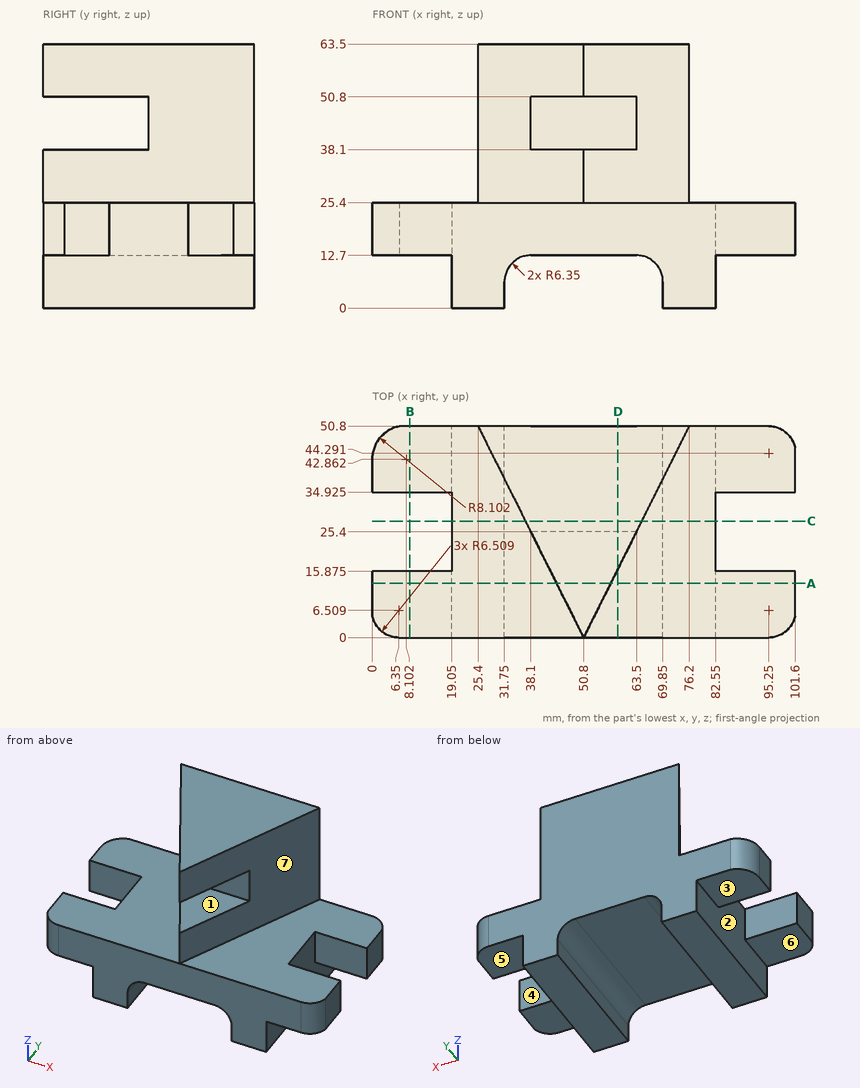
Design review of the part shown in the three views and the two pictorial views. Dimensions are in mm from the part's minimum x, y and z. A direction names the side the tool comes from. Give positions to 0.01 mm unless a question says otherwise; leave off trailing zeros. Loops run counter-clockwise (first coordinate to the right, second up) from the corner with the lowest first, then second, coordinate; pieces in that order, holes last. Notation, with made-up numbers: (11.5, 63.25) - (36.5, 63.25) arc R19 ccw to (36.5, 85.25) - close; hole circle Ø8 at (31.5, -13). An arc over 180 degrees is marked (long way). Answer as a JSON object with one key per item and string values.
Q1. For the marked faces 4, 5, 6 and 7, list the 3-axis set-ups (+Z, -Z, +X, -X, +Y, -Y) from which the entire face can be reached by the end or side of a thin tool; tool diameter is ignored.
Worked out:
{"face 4": "+Z, -Z, +X", "face 5": "-Z, +X, +Y, -Y", "face 6": "-Z, -X, +Y, -Y", "face 7": "+Z, +X, -Y"}
Q2. Add section D-D on x = 59. State the section outline as (y, z) points, plus the area to 3 significant figures.
Worked out:
{"outline": "(0, 12.7) - (50.8, 12.7) - (50.8, 63.5) - (16.4, 63.5) - (16.4, 50.8) - (25.4, 50.8) - (25.4, 38.1) - (16.4, 38.1) - (16.4, 25.4) - (0, 25.4) - close", "area": "1,840 mm^2"}
Q3. Insertion check: pin 1 (17.5 mm diameter, centred on x = 95, y = 44, fed in from -Z); pin 2 (1 mm diameter, centred on x = 24.5, y = 10, fed in from +Z); pin 3 (20.5 mm diameter, centred on x = 47.5, y = 11.5, fed in from -Z); pin 4 (12 mm diameter, centred on x = 68, y = 24, fed in from +Z). Each pin has a flat end and moves straight along its axis. Give the tip position at first contact, or say it passes through.
Worked out:
{"pin 1": "stops at z = 12.7", "pin 2": "stops at z = 25.4", "pin 3": "stops at z = 12.64", "pin 4": "stops at z = 63.5"}
Q4. Add section B-B on x = 9. State the section outline as (y, z) points (1 decimal), plus the area to 3 significant figures.
Worked out:
{"outline": "(0, 12.7) - (15.9, 12.7) - (15.9, 25.4) - (0, 25.4) - close; (34.9, 12.7) - (50.8, 12.7) - (50.8, 25.4) - (34.9, 25.4) - close", "area": "403 mm^2"}
Q5. Mouldability with a two-part tool opening along Z and no side actions: class the marked faces 1, 2 and 3 as +Z half, -Z half, draft (parallel to the pull), parting line (faces both ways), or undercut.
Worked out:
{"face 1": "undercut", "face 2": "draft", "face 3": "-Z half"}
Q6. To check wall thickness, follow line 1 along Y through (x, z) = (7, 19.5) (1 decimal); line 2 along Z through (x, y) = (59.5, 3); line 3 along Z through (x, y) = (70, 4). State the ranges of each line that lie inside material, in increasing order.
Worked out:
{"line 1": "y = 0 to 15.9, 34.9 to 50.8", "line 2": "z = 12.7 to 25.4", "line 3": "z = 0 to 25.4"}
Q7. Add section A-A on y = 13. State the section outline as (x, z) points.
Worked out:
{"outline": "(0, 12.7) - (19.05, 12.7) - (19.05, 0) - (31.75, 0) - (31.75, 6.35) arc R6.35 cw to (38.1, 12.7) - (63.5, 12.7) arc R6.35 cw to (69.85, 6.35) - (69.85, 0) - (82.55, 0) - (82.55, 12.7) - (101.6, 12.7) - (101.6, 25.4) - (57.3, 25.4) - (57.3, 38.1) - (44.3, 38.1) - (44.3, 25.4) - (0, 25.4) - close; (44.3, 50.8) - (57.3, 50.8) - (57.3, 63.5) - (44.3, 63.5) - close"}
Q8. Add section C-C on y = 28. State the section outline as (x, z) points.
Worked out:
{"outline": "(19.05, 0) - (31.75, 0) - (31.75, 6.35) arc R6.35 cw to (38.1, 12.7) - (63.5, 12.7) arc R6.35 cw to (69.85, 6.35) - (69.85, 0) - (82.55, 0) - (82.55, 25.4) - (64.8, 25.4) - (64.8, 63.5) - (36.8, 63.5) - (36.8, 25.4) - (19.05, 25.4) - close"}
